Input: part model. Units: mm. Frame: model coordinates. A direction names the side the tool comes from. Round coordinates to 2 decimals unless told otherwise and drop trailing zeros. Loops run counter-clockwise (first coordinate to the right, second up) from the corner with the lowest first, then second, coordinate; pieces in that order, holes last.
(1) Cut plane C-C, the plane x = 13.25. Output: boundary loops of the cut face in (y, z).
(2) Access query for faces 4 (the face through (-22, -1, 3)), 5 (the face through (6, -30, 22)), 6 (the face through (13, 1, 3)). Directions: +Z, -Z, +X, -X, +Y, -Y. A direction counts if a zero-diameter tool reaches every point of the face in a straight line with its end or side. Return the directions, or none.
(3) Cut plane A-A, the plane y = 20.5. Output: boundary loops of the cut face in (x, z).
(4) First-contact query: pin 1 Ø4.5 at (y, z) = (-33, 11.475) entering from -X; pin 2 Ø3 at (x, y) = (-20, -0.5) entering from +Z; pin 3 Ø3 at (y, z) = (33, 11.475) entering from +X. Flat tips, straight axial feed; report the tip coordinate or a pass-through.
(5) Line query: line 1 (Y direction, x = 13, z = 1); line 2 (Z direction, x = -45, y = -17.5); line 3 (X direction, y = -1, z = 38.5). Output: solid intervals per line, ascending.
(6) Cut plane D-D, the plane y = -33. Output: boundary loops of the cut face in (x, z) (3 decimals), and give its area (3 significant figures).
(7) Cut plane B-B, the plane z = 28.5. Output: boundary loops of the cut face in (x, y), and give its area (3 significant figures).
(8) Draft query along Z for faces 1 (the face through (3.25, -1, 39)), 2 (the face through (6, 1, 41)), 3 (the face through (6.208, 31.048, 32.091)). Return one class per face: released by +Z, released by -Z, zero draft, split by the parting line, or undercut.
from build123d import *

# Parameters (mm, degrees)
CROQUIS2_W                 = 34.5
CROQUIS2_H                 = 80
SALIENTE_EXTRUIR2_DEPTH    = 3
CROQUIS3_W                 = 6
CROQUIS3_H                 = 80
SALIENTE_EXTRUIR3_DEPTH    = 38
CORTAR_EXTRUIR3_DEPTH      = 64.112993908
CORTAR_EXTRUIR3_DEPTH_BACK = 64.112993908
CROQUIS7_W                 = 32
CROQUIS7_H                 = 60
CROQUIS5_R                 = 2
CORTAR_EXTRUIR2_DEPTH      = 61.837899372
CROQUIS8_W                 = 3
CROQUIS8_H                 = 80
SALIENTE_EXTRUIR5_DEPTH    = 30.74
CROQUIS9_R                 = 2
CORTAR_EXTRUIR4_DEPTH      = 30.74
CROQUIS10_R                = 2
CORTAR_EXTRUIR5_DEPTH      = 194


with BuildPart() as part:
    # Croquis2 → Saliente-Extruir2 (new body)
    with BuildSketch(Plane.XY):
        Rectangle(CROQUIS2_W, CROQUIS2_H)
    extrude(amount=SALIENTE_EXTRUIR2_DEPTH)

    # Croquis3 → Saliente-Extruir3 (add)
    with BuildSketch(Plane.XY.offset(3)):
        with Locations((6.25, 0)):
            Rectangle(CROQUIS3_W, CROQUIS3_H)
    extrude(amount=SALIENTE_EXTRUIR3_DEPTH)

    # Croquis7 → Cortar-Extruir3 (cut, two sides: drawn at the far end of the back side and taken through both)
    with BuildSketch(Plane(origin=(9.25, 0, 0), x_dir=(0, 0, -1), z_dir=(1, 0, 0)).offset(-CORTAR_EXTRUIR3_DEPTH_BACK)):
        with Locations((-22, 0)):
            Rectangle(CROQUIS7_W, CROQUIS7_H)
    extrude(amount=CORTAR_EXTRUIR3_DEPTH + CORTAR_EXTRUIR3_DEPTH_BACK, mode=Mode.SUBTRACT)

    # Croquis5 → Cortar-Extruir2 (cut, through all)
    with BuildSketch(Plane.ZY.offset(-3.25)):
        with Locations((11.475, 33)):
            Circle(CROQUIS5_R)
        with Locations((32.525, 33)):
            Circle(CROQUIS5_R)
        with Locations(Location((32.525, -33, 0), (0, 0, 270))):
            Circle(CROQUIS5_R)
        with Locations(Location((11.475, -33, 0), (0, 0, 270))):
            Circle(CROQUIS5_R)
    extrude(amount=-CORTAR_EXTRUIR2_DEPTH, mode=Mode.SUBTRACT)

    # Croquis8 → Saliente-Extruir5 (add)
    with BuildSketch(Plane(origin=(-17.25, -40, 0), x_dir=(0, 0, -1), z_dir=(1, 0, 0))):
        with Locations((-1.5, 40)):
            Rectangle(CROQUIS8_W, CROQUIS8_H)
    extrude(amount=-SALIENTE_EXTRUIR5_DEPTH)

    # Croquis9 → Cortar-Extruir4 (cut)
    with BuildSketch(Plane.XY.offset(3)):
        with Locations((-37.99, 30)):
            Circle(CROQUIS9_R)
        with Locations((-37.99, -30)):
            Circle(CROQUIS9_R)
    extrude(amount=-CORTAR_EXTRUIR4_DEPTH, mode=Mode.SUBTRACT)

    # Croquis10 → Cortar-Extruir5 (cut)
    with BuildSketch(Plane.XY.offset(3)):
        with Locations((13.25, 30)):
            Circle(CROQUIS10_R)
        with Locations((13.25, -30)):
            Circle(CROQUIS10_R)
    extrude(amount=-CORTAR_EXTRUIR5_DEPTH, mode=Mode.SUBTRACT)


solid = part.part
Reported:
1. outline: (-40, 0) - (-32, 0) - (-32, 3) - (-40, 3) - close; (-28, 0) - (28, 0) - (28, 3) - (-28, 3) - close; (32, 0) - (40, 0) - (40, 3) - (32, 3) - close
2. face 4: +Z, -X, +Y, -Y
2. face 5: +X, -X
2. face 6: +Z, +X, +Y, -Y
3. outline: (-47.99, 0) - (17.25, 0) - (17.25, 3) - (9.25, 3) - (9.25, 6) - (3.25, 6) - (3.25, 3) - (-47.99, 3) - close; (3.25, 38) - (9.25, 38) - (9.25, 41) - (3.25, 41) - close
4. pin 1: stops at x = 3.25
4. pin 2: stops at z = 3
4. pin 3: passes through
5. line 1: y = -40 to -31.98, -28.02 to 28.02, 31.98 to 40
5. line 2: z = 0 to 3
5. line 3: x = 3.25 to 9.25
6. outline: (-47.99, 0) - (17.25, 0) - (17.25, 3) - (9.25, 3) - (9.25, 9.475) - (3.25, 9.475) - (3.25, 3) - (-47.99, 3) - close; (3.25, 13.475) - (9.25, 13.475) - (9.25, 30.525) - (3.25, 30.525) - close; (3.25, 34.525) - (9.25, 34.525) - (9.25, 41) - (3.25, 41) - close
6. area: 376 mm2
7. outline: (3.25, -40) - (9.25, -40) - (9.25, -30) - (3.25, -30) - close; (3.25, 30) - (9.25, 30) - (9.25, 40) - (3.25, 40) - close
7. area: 120 mm2
8. face 1: zero draft
8. face 2: released by +Z
8. face 3: undercut
